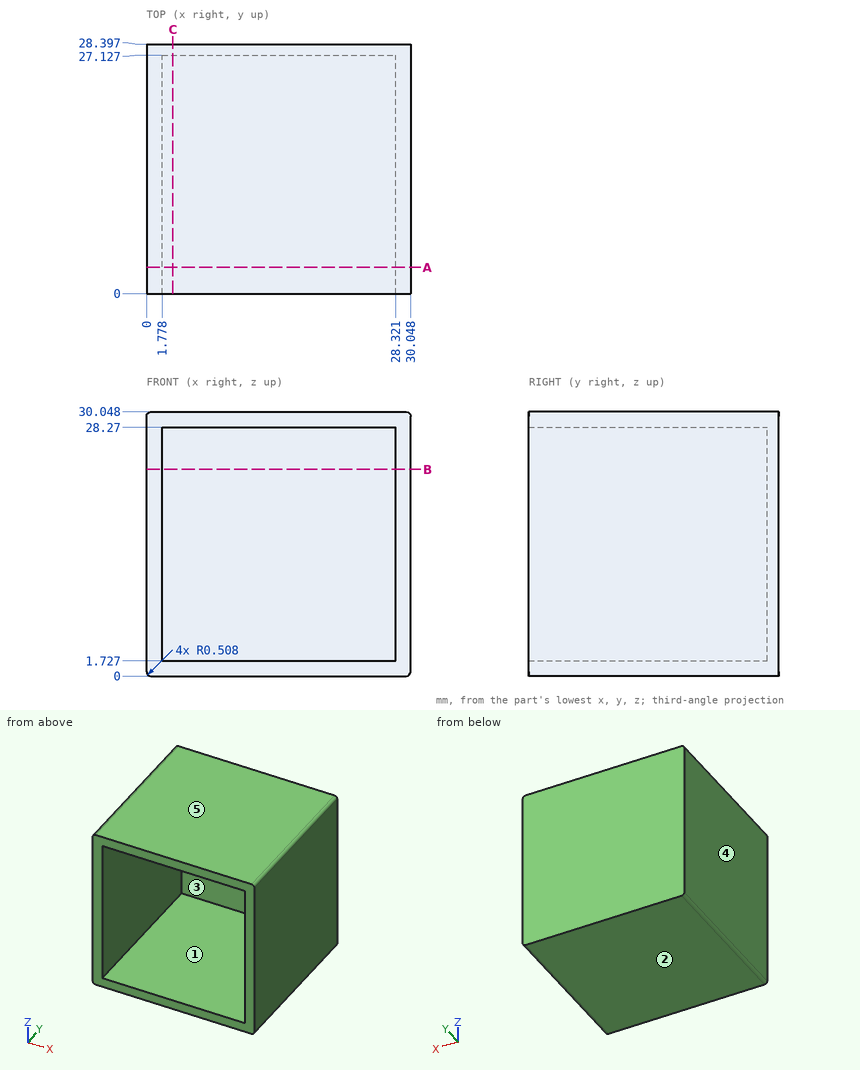
Study the drawing (mm; zero at the part's minimum x, y, z) and answer. A direction names the side the tool comes from. Coordinates: 2 decimals unless noted, no trailing zeros. Write each loop counter-clockwise with the first axis right and the second up, starting at its lowest first coordinate (ties: lowest second). Pieces come first, ordered by that corner, then holes.
Q1. A cutting plane is placed at C-C, the plane x = 3. Give the vertices of the cut face in (y, z).
Q2. Which of the six approach directions +Z, -Z, +X, -X, +Y, -Y give full straight-line access (tool end or side, diameter ignored) to the marked faces 1 and 2?
Q3. This flat-tipped pin is pushed along its axis until it touches: pin 1 Ø6 at (x, z) = (24, 18) entering from -Y. Where does it stop, or does it pass through?
Q4. Determine the mould class of the marked faces 3, 4 and 5 for opening direction Z: released by +Z, released by -Z, zero draft, split by the parting line, or undercut.
Q5. Find the intervals of material crossed by line 1 (Z direction, x = 25.5, y = 9.75); line 2 (X direction, y = 24.25, z = 3.5); line 3 (Y direction, x = 28, z = 17.5), in increasing order.
Q6. A cutting plane is placed at B-B, the plane z = 23.5. Give the vertices of the cut face in (x, y), then the cut area to 3 significant figures.
Q7. A cutting plane is placed at A-A, the plane y = 3. Give the vertices of the cut face in (x, z).
Findings below:
1. outline: (0, 0) - (28.4, 0) - (28.4, 30.05) - (0, 30.05) - (0, 28.27) - (27.13, 28.27) - (27.13, 1.73) - (0, 1.73) - close
2. face 1: -Y
2. face 2: -Z, +X, -X, +Y, -Y
3. pin 1: stops at y = 27.13
4. face 3: undercut
4. face 4: zero draft
4. face 5: released by +Z
5. line 1: z = 0 to 1.73, 28.27 to 30.05
5. line 2: x = 0 to 1.78, 28.32 to 30.05
5. line 3: y = 27.13 to 28.4
6. outline: (0, 0) - (1.78, 0) - (1.78, 27.13) - (28.32, 27.13) - (28.32, 0) - (30.05, 0) - (30.05, 28.4) - (0, 28.4) - close
6. area: 133 mm2
7. outline: (0, 0.51) arc R0.51 ccw to (0.51, 0) - (29.54, 0) arc R0.51 ccw to (30.05, 0.51) - (30.05, 29.54) arc R0.51 ccw to (29.54, 30.05) - (0.51, 30.05) arc R0.51 ccw to (0, 29.54) - close; hole (1.78, 1.73) - (28.32, 1.73) - (28.32, 28.27) - (1.78, 28.27) - close
